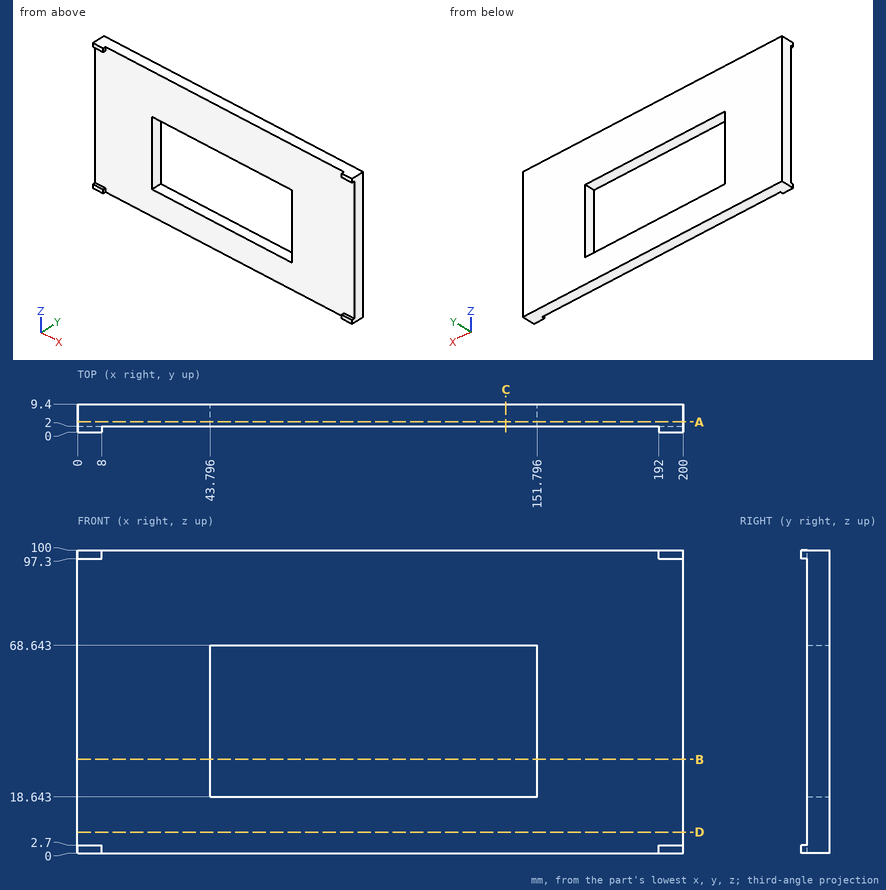
Drawing for the job (mm, zero at the part's lowest x, y, z). Round coordinates to 2 decimals unless told otherwise and drop trailing zeros. Loops run counter-clockwise (first coordinate to the right, second up) from the corner with the lowest first, then second, coordinate; pieces in that order, holes last. Notation, with made-up numbers: (84.5, 12) - (112.5, 12) arc R17 cw to (112.5, 32) - close; hole circle Ø4 at (24, 19.25). An arc over 180 degrees is marked (long way). Write each question's results on one line, items separated by ' | '.
(1) Saw through at C-C, the plane x = 141.5. List the corners of the cut face in (y, z), then the cut area to 3 significant figures.
Answer below:
outline: (2, 0) - (9.4, 0) - (9.4, 18.64) - (2, 18.64) - close; (2, 68.64) - (9.4, 68.64) - (9.4, 100) - (2, 100) - close | area: 370 mm^2
(2) Saw through at B-B, the plane z = 31. List the corners of the cut face in (x, y).
Answer below:
outline: (0, 2) - (43.8, 2) - (43.8, 9.4) - (0, 9.4) - close; (151.8, 2) - (200, 2) - (200, 9.4) - (151.8, 9.4) - close
(3) Saw through at A-A, the plane y = 3.5. List the corners of the cut face in (x, z).
Answer below:
outline: (0, 0) - (200, 0) - (200, 100) - (0, 100) - close; hole (43.8, 18.64) - (151.8, 18.64) - (151.8, 68.64) - (43.8, 68.64) - close
(4) Wall check: L1, parallel to Z at x = 74, y = 9.25; L2, parallel to X at y = 4.5, z = 39.5; L3, parallel to Y at x = 186, z = 89.5. Give the ranges that are in metal, low to high.
Answer below:
L1: z = 0 to 18.64, 68.64 to 100 | L2: x = 0 to 43.8, 151.8 to 200 | L3: y = 2 to 9.4
(5) Saw through at D-D, the plane z = 7. List the corners of the cut face in (x, y).
Answer below:
outline: (0, 2) - (200, 2) - (200, 9.4) - (0, 9.4) - close
